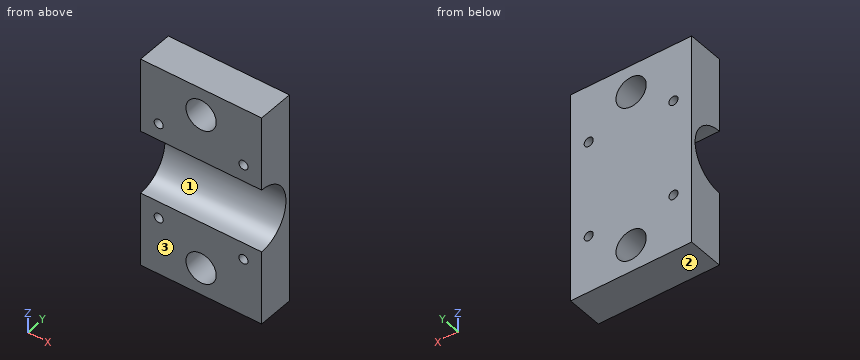
```python
from build123d import *

# Parameters (mm, degrees)
F0_W     = 40
F0_H     = 70
F0_R     = 1.5
F0_R_2   = 5
F1_DEPTH = 12
F3_DEPTH = 40.001


with BuildPart() as f1:
    # F0 (on Front) → F1 (new body)
    with BuildSketch(Plane.XZ):
        with Locations((20, 35)):
            Rectangle(F0_W, F0_H)
        with Locations((6, 19)):
            Circle(F0_R, mode=Mode.SUBTRACT)
        with Locations((20, 9)):
            Circle(F0_R_2, mode=Mode.SUBTRACT)
        with Locations((34, 19)):
            Circle(F0_R, mode=Mode.SUBTRACT)
        with Locations((6, 51)):
            Circle(F0_R, mode=Mode.SUBTRACT)
        with Locations((34, 51)):
            Circle(F0_R, mode=Mode.SUBTRACT)
        with Locations((20, 61)):
            Circle(F0_R_2, mode=Mode.SUBTRACT)
    extrude(amount=F1_DEPTH)

    # F2 (on face) → F3 (cut, through all)
    with BuildSketch(Plane.YZ.offset(40)):
        with BuildLine():
            ThreePointArc((-12, 24.5), (-1.5, 35), (-12, 45.5))
            Line((-12, 45.5), (-12, 24.5))
        make_face()
    extrude(amount=-F3_DEPTH, mode=Mode.SUBTRACT)


solid = f1.part
```
Check sheet for the modelled part. Datum: model origin and axes. Units: mm. Face numbers are marked on the shaded views. Coordinates: 2 decimals unless noted, no trailing zeros. Order: outer loops, then holes, each group sorted by start corner. A loop starts at its lowest first (then second) coordinate and runs counter-clockwise, first axis right, second up. Notation, with made-up numbers: M -38,-21 L 9,-21 A19 cw 9,4 Z; hole C 48,-28.5 d8. An arc over 180 degrees is marked long. Write each question's results on one line, items separated by ' | '. Start each with the question number.
1. Cross-section at B-B on x = 34. Record the cut outline in (y, z).
2. Cross-section at A-A on y = -7. Record the cut outline in (x, z), and give its area (3 significant figures).
3. Mould release check, pull along Z, two halves, no side actions. Record for the marked faces 1, 2 and 3: +Z half, -Z half, draft (parallel to the pull), parting line (faces both ways), or undercut.
4. Go/stop test with a flat-tipped pin: P1, Ø5, axis at x = 11, z = 42, coming from the -Y side. Record where the tip stops, or that it passes through.
5. Cross-section at C-C on z = 19. Record the cut outline in (x, y).
6. Cross-section at D-D on z = 9. Record the cut outline in (x, y), and give its area (3 significant figures).
7. Material ranges on probe 1 along Z at (x, y) = (6, -3.75); probe 2 along Z at (x, y) = (6.5, -9); probe 3 along Z at (x, y) = (31, -3.25), recorded low to high.
Checks:
1) outline: M -12,0 L 0,0 L 0,17.5 L -12,17.5 Z; M -12,20.5 L 0,20.5 L 0,49.5 L -12,49.5 L -12,45.5 A10.5 cw -12,24.5 Z; M -12,52.5 L 0,52.5 L 0,70 L -12,70 Z
2) outline: M 0,0 L 40,0 L 40,25.77 L 0,25.77 Z; M 0,44.23 L 40,44.23 L 40,70 L 0,70 Z; hole C 6,19 d3; hole C 6,51 d3; hole C 20,9 d10; hole C 20,61 d10; hole C 34,19 d3; hole C 34,51 d3 | area: 1,880 mm²
3) face 1: undercut | face 2: -Z half | face 3: draft
4) P1: stops at y = -7.53
5) outline: M 0,-12 L 4.5,-12 L 4.5,0 L 0,0 Z; M 7.5,-12 L 32.5,-12 L 32.5,0 L 7.5,0 Z; M 35.5,-12 L 40,-12 L 40,0 L 35.5,0 Z
6) outline: M 0,-12 L 15,-12 L 15,0 L 0,0 Z; M 25,-12 L 40,-12 L 40,0 L 25,0 Z | area: 360 mm²
7) probe 1: z = 0 to 17.5, 20.5 to 28.5, 41.5 to 49.5, 52.5 to 70 | probe 2: z = 0 to 17.59, 20.41 to 24.94, 45.06 to 49.59, 52.41 to 70 | probe 3: z = 0 to 29.2, 40.8 to 70
